from build123d import *

# Parameters (mm, degrees)
SKETCH1_R           = 2.4892
SKETCH1_W           = 16.49984
SKETCH1_H           = 16.49984
BOSS_EXTRUDE1_DEPTH = 5.08
CUT_EXTRUDE1_DEPTH  = 11.16
SKETCH4_R           = 20.0025
SKETCH4_R_2         = 11.58875
CUT_EXTRUDE2_DEPTH  = 2.3495
SKETCH6_R           = 1.651
CUT_EXTRUDE3_DEPTH  = 11.16
FILLET1_R           = 0.762
FILLET2_R           = 3.175
FILLET3_R           = 2.54


with BuildPart() as part:
    # Sketch1 → Boss-Extrude1 (new body, symmetric)
    with BuildSketch(Plane(origin=(0, 0, 0), x_dir=(1, 0, 0), z_dir=(0, 1, 0))):
        with BuildLine():
            ThreePointArc((-4.56242174, 13.874088542), (0, 20.0025), (4.56242174, 13.874088542))
            ThreePointArc((4.56242174, 13.874088542), (14.605, 0), (4.56242174, -13.874088542))
            ThreePointArc((4.56242174, -13.874088542), (0, -20.0025), (-4.56242174, -13.874088542))
            ThreePointArc((-4.56242174, -13.874088542), (-14.605, 0), (-4.56242174, 13.874088542))
        make_face()
        with Locations((0, 15.24)):
            Circle(SKETCH1_R, mode=Mode.SUBTRACT)
        with Locations((0, -15.24)):
            Circle(SKETCH1_R, mode=Mode.SUBTRACT)
        Rectangle(SKETCH1_W, SKETCH1_H, mode=Mode.SUBTRACT)
    extrude(amount=BOSS_EXTRUDE1_DEPTH, both=True)

    # Sketch2 → Cut-Extrude1 (cut, through all)
    with BuildSketch(Plane(origin=(0, 5.08, 0), x_dir=(1, 0, 0), z_dir=(0, 1, 0))):
        with BuildLine():
            Line((-11.43, -9.091816375), (-11.43, 9.091816375))
            ThreePointArc((-11.43, 9.091816375), (-14.605, 0), (-11.43, -9.091816375))
        make_face()
        with BuildLine():
            Line((11.43, -9.091816375), (11.43, 9.091816375))
            ThreePointArc((11.43, 9.091816375), (14.605, 0), (11.43, -9.091816375))
        make_face()
    extrude(amount=-CUT_EXTRUDE1_DEPTH, mode=Mode.SUBTRACT)

    # Sketch4 → Cut-Extrude2 (cut)
    with BuildSketch(Plane(origin=(0, 5.08, 0), x_dir=(1, 0, 0), z_dir=(0, 1, 0))):
        Circle(SKETCH4_R)
        Circle(SKETCH4_R_2, mode=Mode.SUBTRACT)
    extrude(amount=-CUT_EXTRUDE2_DEPTH, mode=Mode.SUBTRACT)

    # Sketch6 → Cut-Extrude3 (cut, through all)
    with BuildSketch(Plane(origin=(0, 5.08, 0), x_dir=(1, 0, 0), z_dir=(0, 1, 0))):
        with Locations((-7.082486704, 7.082486704)):
            Circle(SKETCH6_R)
        with Locations((7.135507627, 7.031771379)):
            Circle(SKETCH6_R)
        with Locations((7.082486704, -7.082486704)):
            Circle(SKETCH6_R)
        with Locations((-7.078544383, -7.086442383)):
            Circle(SKETCH6_R)
    extrude(amount=-CUT_EXTRUDE3_DEPTH, mode=Mode.SUBTRACT)

    # Fillet1
    fillet1_edges = [part.edges().sort_by_distance(p)[0] for p in [
        (-8.567823829, 3.90525, -7.803301954),
        (7.861200497, 3.90525, -8.514731547),
        (7.803301954, 3.90525, 8.567823829),
        (-7.798496392, 3.90525, 8.572198119),
        (-8.563496345, 3.90525, 7.808050776),
        (8.567823829, 3.90525, 7.803301954),
        (8.628935612, 3.90525, -7.735670415),
        (-7.803301954, 3.90525, -8.567823829),
    ]]
    fillet(fillet1_edges, radius=FILLET1_R)

    # Fillet2
    fillet2_edges = [part.edges().sort_by_distance(p)[0] for p in [
        (-4.56242174, -1.17475, -13.874088542),
        (4.56242174, -1.17475, -13.874088542),
        (4.56242174, -1.17475, 13.874088542),
        (-4.56242174, -1.17475, 13.874088542),
    ]]
    fillet(fillet2_edges, radius=FILLET2_R)

    # Fillet3
    fillet3_edges = [part.edges().sort_by_distance(p)[0] for p in [
        (-11.43, -1.17475, 9.091816375),
        (-11.43, -1.17475, -9.091816375),
        (11.43, -1.17475, -9.091816375),
        (11.43, -1.17475, 9.091816375),
    ]]
    fillet(fillet3_edges, radius=FILLET3_R)


solid = part.part
For this review, take the finished solid that the model builds, in its own axes (mm). A direction names the side the tool comes from. Give positions to 0.01 mm unless a question says otherwise; leave off trailing zeros. Order: outer loops, then holes, each group sorted by start corner. A loop starts at its lowest first (then second) coordinate and runs counter-clockwise, first axis right, second up. Notation, with made-up numbers: (1.5, -20) - (9.5, -20) arc R27 ccw to (9.5, 15) - close; hole circle Ø1 at (7.25, 18). An arc over 180 degrees is marked (long way). Answer as a JSON object with one key per item and string values. Group by question number.
Item 1: Take a section at D-D on y = 1.5. Give the number of separate pieces and of enclosed holes in the cut face, and give its area (3 significant figures).
Item 2: Machinability: for faces 4 (the flat face through (0, 5.08, 10)), 5 (the cylindrical face through (-10.83, 3.92, 4.12)), 6 (the cylindrical face through (-0.09, 3.92, 11.59)), which of the approach directions +Z, -Z, +X, -X, +Y, -Y give a long, thin tool a straight path to every point of the face, cutting with its end or side? Answer none if there is none.
Item 3: Take a section at B-B on z = 1. Give the boundary of the cut face in (x, y), and give its area (3 significant figures).
Item 4: Take a section at A-A on x = 0. Give the boundary of the cut face in (y, z).
Item 5: Wall thickness on line 1 along Z through (x, y) = (0, -2.25); line 2 along X through (y, z) = (-2.5, 3.5); line 3 along X through (y, z) = (0.5, 15.24): over which ranges is each line inside the solid? List them lowest first.
Item 6: Clearance check with flat-ended pins moving along their axes: pin 1 Ø1 at (y, z) = (4, 4.5) entering from +X; pin 2 Ø1.5 at (x, y) = (6.5, 3) entering from -Z; pin 3 Ø3 at (x, y) = (-2, 2.5) entering from -Z. State where each tip first meets the part, or that it passes through.
Item 7: Draft analysis for pull direction X (two halves, no side actions). For faces 1 (the cylindrical face through (1.149, -1.229, 17.448)), 2 (the cylindrical face through (8.81, -1.12, 11.65)), 3 (the cylindrical face through (0.1, -1.1, 20)), state which applies: pulls with the +X half, pulls with the -X half, needs draft (parallel to the pull), parting line crosses it, or undercut.
Item 8: Take a section at C-C on x = -7.5. Give the boundary of the cut face in (y, z), and give its area (3 significant figures).
Reported:
{
 "1": {"separate pieces": "1", "enclosed holes": "3", "area": "365 mm^2"},
 "2": {"face 4": "+Z, -Z, +X, -X, +Y", "face 5": "+Z, -X, +Y", "face 6": "+Z, +Y"},
 "3": {"outline": "(-11.43, -5.08) - (-8.25, -5.08) - (-8.25, 5.08) - (-11.43, 5.08) - close; (8.25, -5.08) - (11.43, -5.08) - (11.43, 5.08) - (8.25, 5.08) - close", "area": "64.6 mm^2"},
 "4": {"outline": "(-5.08, -20) - (2.73, -20) - (2.73, -17.73) - (-5.08, -17.73) - close; (-5.08, -12.75) - (2.73, -12.75) - (2.73, -11.59) - (5.08, -11.59) - (5.08, -8.25) - (-5.08, -8.25) - close; (-5.08, 8.25) - (5.08, 8.25) - (5.08, 11.59) - (2.73, 11.59) - (2.73, 12.75) - (-5.08, 12.75) - close; (-5.08, 17.73) - (2.73, 17.73) - (2.73, 20) - (-5.08, 20) - close"},
 "5": {"line 1": "-20 to -17.73, -12.75 to -8.25, 8.25 to 12.75, 17.73 to 20", "line 2": "-11.43 to -8.25, 8.25 to 11.43", "line 3": "-4.81 to -2.49, 2.49 to 4.81"},
 "6": {"pin 1": "x = 10.88", "pin 2": "z = -13.55", "pin 3": "z = -19.98"},
 "7": {"face 1": "undercut", "face 2": "pulls with the +X half", "face 3": "parting line crosses it"},
 "8": {"outline": "(-5.08, -12.53) - (2.73, -12.53) - (2.73, -8.68) - (-5.08, -8.68) - close; (-5.08, 8.68) - (2.73, 8.68) - (2.73, 12.53) - (-5.08, 12.53) - close", "area": "60.2 mm^2"}
}
